from build123d import *

# Parameters (mm, degrees)
F0_W     = 12.7
F0_H     = 7.62
F0_W_2   = 6.1468
F0_H_2   = 12.7
F1_DEPTH = 7.62
F2_R     = 25.4
F3_DEPTH = 25.4
F5_DEPTH = 25.4
F6_R     = 5.08


with BuildPart() as f1:
    # F0 (on Top) → F1 (new body)
    with BuildSketch(Plane.XY):
        Polygon((-69.044474, 45.180961), (-69.044474, 50.260961), (-81.744474, 50.260961), (-81.744474, 27.400961), (-69.044474, 27.400961), (-69.044474, 32.480961), (-75.191274, 32.480961), (-75.191274, 45.180961), align=None)
        Polygon((-56.344474, 57.880961), (-69.044474, 57.880961), (-69.044474, 50.260961), (-69.044474, 45.180961), (-62.491274, 45.180961), (-56.344474, 45.180961), (-56.344474, 50.260961), align=None)
        with Locations((-49.994474, 54.070961)):
            Rectangle(F0_W, F0_H)
        with Locations((-49.994474, 23.590961)):
            Rectangle(F0_W, F0_H)
        Polygon((-56.344474, 27.400961), (-56.344474, 32.480961), (-62.491274, 32.480961), (-69.044474, 32.480961), (-69.044474, 27.400961), (-69.044474, 19.780961), (-56.344474, 19.780961), align=None)
        with Locations((-59.417874, 38.830961)):
            Rectangle(F0_W_2, F0_H_2)
    extrude(amount=F1_DEPTH)


with BuildPart() as f3:
    # F2 (on Top) → F3 (new body)
    with BuildSketch(Plane.XY):
        with Locations((41.206498, 17.812403)):
            Circle(F2_R)
    extrude(amount=F3_DEPTH)


with BuildPart() as f5:
    # F4 (on Top) → F5 (new body)
    with BuildSketch(Plane.XY):
        Polygon((42.736534, 52.771983), (27.891826, 63.671286), (25.875106, 45.36574), align=None)
    extrude(amount=F5_DEPTH)

    # F6
    f6_edges = [f5.edges().sort_by_distance(p)[0] for p in [
        (35.31418, 58.221634, 25.4),
        (26.883466, 54.518513, 25.4),
        (34.30582, 49.068861, 25.4),
        (35.31418, 58.221634, 0),
        (26.883466, 54.518513, 0),
        (34.30582, 49.068861, 0),
    ]]
    fillet(f6_edges, radius=F6_R)


solid = f1.part
Geometry check sheet. Reference: the model listing, model coordinates, mm. A direction names the side the tool comes from. Give positions to 0.01 mm unless a question says otherwise; leave off trailing zeros. Order: outer loops, then holes, each group sorted by start corner. A loop starts at its lowest first (then second) coordinate and runs counter-clockwise, first axis right, second up.
1. Sectioned sample at B-B (y = 42). Record the boundary of the cut face in (x, z), then the cut area to 3 significant figures.
Completed:
outline: (-81.74, 0) - (-75.19, 0) - (-75.19, 7.62) - (-81.74, 7.62) - close; (-62.49, 0) - (-56.34, 0) - (-56.34, 7.62) - (-62.49, 7.62) - close
area: 96.8 mm2
2. Sectioned sample at A-A (x = -65). Record the boundary of the cut face in (y, z), then the cut area to 3 significant figures.
Completed:
outline: (19.78, 0) - (32.48, 0) - (32.48, 7.62) - (19.78, 7.62) - close; (45.18, 0) - (57.88, 0) - (57.88, 7.62) - (45.18, 7.62) - close
area: 194 mm2
3. Draft check along Y on faces 4 (the face through (-50, 50.261, 4)), 5 (the face through (-75, 27.401, 4)), 6 (the face through (-56, 57.881, 4)). Enter one of: pulls with the +Y half, pulls with the -Y half, needs draft (parallel to the pull), parting line crosses it, or undercut.
Completed:
face 4: undercut
face 5: pulls with the -Y half
face 6: pulls with the +Y half
4. Access from +Z, -Z, +X, -X, +Y, -Y to the whole of each face (thin tool, end or side, straight path). Record for faces 1 (the face through (-75, 50.261, 4)), 2 (the face through (-75.191, 39, 4)), 3 (the face through (-56.344, 39, 4)).
Completed:
face 1: +Z, -Z, -X, +Y
face 2: +Z, -Z
face 3: +Z, -Z, +X
5. Sectioned sample at D-D (y = 32). Record the boundary of the cut face in (x, z).
Completed:
outline: (-81.74, 0) - (-56.34, 0) - (-56.34, 7.62) - (-81.74, 7.62) - close
6. Depth check by flat-ended pin: pin 1 (2.5 mm diameter, centred on y = 42.5, z = 2, fed in from +X); pin 2 (3 mm diameter, centred on x = -70.5, z = 3, fed in from -Y); pin 3 (2.5 mm diameter, centred on y = 24.5, z = 3, fed in from -X); pin 4 (2.5 mm diameter, centred on x = -75, z = 3.5, fed in from -Y). Enter the tip coordinate at first touch or a pass-through.
Completed:
pin 1: stops at x = -56.34
pin 2: stops at y = 19.78
pin 3: stops at x = -69.04
pin 4: stops at y = 27.4
7. Scan lines: line 1 (Y direction, x = -65.5, z = 5.75); line 2 (Y direction, x = -53, z = 2.5); line 3 (X direction, y = 34, z = 6.25). Record each from-to range of solid material in increasing order.
Completed:
line 1: y = 19.78 to 32.48, 45.18 to 57.88
line 2: y = 19.78 to 27.4, 50.26 to 57.88
line 3: x = -81.74 to -75.19, -62.49 to -56.34
8. Sectioned sample at C-C (z = 6.75). Record the boundary of the cut face in (x, y).
Completed:
outline: (-81.74, 27.4) - (-69.04, 27.4) - (-69.04, 19.78) - (-43.64, 19.78) - (-43.64, 27.4) - (-56.34, 27.4) - (-56.34, 50.26) - (-43.64, 50.26) - (-43.64, 57.88) - (-69.04, 57.88) - (-69.04, 50.26) - (-81.74, 50.26) - close; hole (-75.19, 32.48) - (-62.49, 32.48) - (-62.49, 45.18) - (-75.19, 45.18) - close
